```python
from build123d import *

# Parameters (mm, degrees)
F0_W      = 127
F0_H      = 127
F1_DEPTH  = 127
F2_R      = 10.16
F3_R      = 11.0292636168
F4_DEPTH  = 5.08
F6_DEPTH  = 5.08
F7_R      = 8.89
F8_DEPTH  = 5.08
F9_R      = 11.176
F10_DEPTH = 5.08
F12_DEPTH = 5.08
F14_DEPTH = 5.08


with BuildPart() as f1:
    # F0 (on Top) → F1 (new body)
    with BuildSketch(Plane.XY):
        with Locations((-72.0648214515, 42.2182492242)):
            Rectangle(F0_W, F0_H)
    extrude(amount=F1_DEPTH)

    # F2
    f2_edges = [f1.edges().sort_by_distance(p)[0] for p in [
        (-135.564821, -21.281751, 63.5),
        (-8.564821, -21.281751, 63.5),
        (-72.064821, -21.281751, 0),
        (-72.064821, -21.281751, 127),
        (-72.064821, 105.718249, 127),
        (-135.564821, 42.218249, 127),
        (-8.564821, 42.218249, 127),
        (-135.564821, 105.718249, 63.5),
        (-135.564821, 42.218249, 0),
        (-8.564821, 105.718249, 63.5),
        (-72.064821, 105.718249, 0),
        (-8.564821, 42.218249, 0),
    ]]
    fillet(f2_edges, radius=F2_R)

    # F3 (on face) → F4 (cut)
    with BuildSketch(Plane(origin=(0, 0, 0), x_dir=(1, 0, 0), z_dir=(0, 0, -1))):
        with Locations((-72.0648214515, -42.2182492242)):
            Circle(F3_R)
    extrude(amount=-F4_DEPTH, mode=Mode.SUBTRACT)

    # F5 (on face) → F6 (cut)
    with BuildSketch(Plane.XY.offset(127)):
        with BuildLine():
            Line((-100.0048214515, 61.2682492242), (-100.0048214515, 79.0482492242))
            ThreePointArc((-100.0048214515, 79.0482492242), (-108.8948214515, 70.1582492242), (-100.0048214515, 61.2682492242))
        make_face()
        with BuildLine():
            ThreePointArc((-91.1148214515, 70.1582492242), (-93.7186421668, 76.444428509), (-100.0048214515, 79.0482492242))
            Line((-100.0048214515, 79.0482492242), (-100.0048214515, 61.2682492242))
            ThreePointArc((-100.0048214515, 61.2682492242), (-93.7186421668, 63.8720699395), (-91.1148214515, 70.1582492242))
        make_face()
        with BuildLine():
            ThreePointArc((-100.0048214515, 53.6482492242), (-108.8948214515, 44.7582492242), (-100.0048214515, 35.8682492242))
            Line((-100.0048214515, 35.8682492242), (-100.0048214515, 53.6482492242))
        make_face()
        with BuildLine():
            Line((-100.0048214515, 53.6482492242), (-100.0048214515, 35.8682492242))
            ThreePointArc((-100.0048214515, 35.8682492242), (-93.7186421668, 38.4720699395), (-91.1148214515, 44.7582492242))
            ThreePointArc((-91.1148214515, 44.7582492242), (-93.7186421668, 51.044428509), (-100.0048214515, 53.6482492242))
        make_face()
        with BuildLine():
            Line((-44.1248214515, 61.2682492242), (-44.1248214515, 79.0482492242))
            ThreePointArc((-44.1248214515, 79.0482492242), (-53.0148214515, 70.1582492242), (-44.1248214515, 61.2682492242))
        make_face()
        with BuildLine():
            ThreePointArc((-35.2348214515, 70.1582492242), (-37.8386421668, 76.444428509), (-44.1248214515, 79.0482492242))
            Line((-44.1248214515, 79.0482492242), (-44.1248214515, 61.2682492242))
            ThreePointArc((-44.1248214515, 61.2682492242), (-37.8386421668, 63.8720699395), (-35.2348214515, 70.1582492242))
        make_face()
        with BuildLine():
            ThreePointArc((-44.1248214515, 53.6482492242), (-53.0148214515, 44.7582492242), (-44.1248214515, 35.8682492242))
            Line((-44.1248214515, 35.8682492242), (-44.1248214515, 53.6482492242))
        make_face()
        with BuildLine():
            Line((-44.1248214515, 53.6482492242), (-44.1248214515, 35.8682492242))
            ThreePointArc((-44.1248214515, 35.8682492242), (-37.8386421668, 38.4720699395), (-35.2348214515, 44.7582492242))
            ThreePointArc((-35.2348214515, 44.7582492242), (-37.8386421668, 51.044428509), (-44.1248214515, 53.6482492242))
        make_face()
        with BuildLine():
            ThreePointArc((-100.0048214515, 28.2482492242), (-108.8948214515, 19.3582492242), (-100.0048214515, 10.4682492242))
            Line((-100.0048214515, 10.4682492242), (-100.0048214515, 28.2482492242))
        make_face()
        with BuildLine():
            Line((-100.0048214515, 28.2482492242), (-100.0048214515, 10.4682492242))
            ThreePointArc((-100.0048214515, 10.4682492242), (-93.7186421668, 13.0720699395), (-91.1148214515, 19.3582492242))
            ThreePointArc((-91.1148214515, 19.3582492242), (-93.7186421668, 25.644428509), (-100.0048214515, 28.2482492242))
        make_face()
        with BuildLine():
            ThreePointArc((-44.1248214515, 28.2482492242), (-53.0148214515, 19.3582492242), (-44.1248214515, 10.4682492242))
            Line((-44.1248214515, 10.4682492242), (-44.1248214515, 28.2482492242))
        make_face()
        with BuildLine():
            Line((-44.1248214515, 28.2482492242), (-44.1248214515, 10.4682492242))
            ThreePointArc((-44.1248214515, 10.4682492242), (-37.8386421668, 13.0720699395), (-35.2348214515, 19.3582492242))
            ThreePointArc((-35.2348214515, 19.3582492242), (-37.8386421668, 25.644428509), (-44.1248214515, 28.2482492242))
        make_face()
    extrude(amount=-F6_DEPTH, mode=Mode.SUBTRACT)

    # F7 (on face) → F8 (cut)
    with BuildSketch(Plane(origin=(-135.5648214515, 0, 0), x_dir=(0, -1, 0), z_dir=(-1, 0, 0))):
        with Locations((-68.8882492242, 90.17)):
            Circle(F7_R)
        with Locations((-68.8882492242, 36.83)):
            Circle(F7_R)
        with Locations((-15.5482492242, 36.83)):
            Circle(F7_R)
        with Locations((-15.5482492242, 90.17)):
            Circle(F7_R)
    extrude(amount=-F8_DEPTH, mode=Mode.SUBTRACT)

    # F9 (on face) → F10 (cut)
    with BuildSketch(Plane.YZ.offset(-8.5648214515)):
        with Locations((6.6322155756, 99.0860336486)):
            Circle(F9_R)
        with Locations((77.8042828729, 27.9139663514)):
            Circle(F9_R)
        with Locations((42.2182492242, 63.5)):
            Circle(F9_R)
    extrude(amount=-F10_DEPTH, mode=Mode.SUBTRACT)

    # F11 (on face) → F12 (cut)
    with BuildSketch(Plane.XZ.offset(21.2817507758)):
        with BuildLine():
            ThreePointArc((-99.8604116578, 102.4715902063), (-106.7595416177, 112.7968678616), (-118.9390370444, 110.3742155928))
            Line((-118.9390370444, 110.3742155928), (-103.1337862713, 94.5689648197))
            ThreePointArc((-103.1337862713, 94.5689648197), (-100.7111340025, 98.1947201662), (-99.8604116578, 102.4715902063))
        make_face()
        with BuildLine():
            ThreePointArc((-40.9958566318, 32.4310351803), (-40.9958566318, 16.6257844072), (-25.1906058587, 16.6257844072))
            Line((-25.1906058587, 16.6257844072), (-40.9958566318, 32.4310351803))
        make_face()
        with BuildLine():
            Line((-40.9958566318, 32.4310351803), (-25.1906058587, 16.6257844072))
            ThreePointArc((-25.1906058587, 16.6257844072), (-22.7679535899, 20.2515397536), (-21.9172312452, 24.5284097937))
            ThreePointArc((-21.9172312452, 24.5284097937), (-28.8163612051, 34.8536874491), (-40.9958566318, 32.4310351803))
        make_face()
        with BuildLine():
            ThreePointArc((-103.1337862713, 32.4310351803), (-118.9390370444, 32.4310351803), (-118.9390370444, 16.6257844072))
            Line((-118.9390370444, 16.6257844072), (-103.1337862713, 32.4310351803))
        make_face()
        with BuildLine():
            Line((-103.1337862713, 32.4310351803), (-118.9390370444, 16.6257844072))
            ThreePointArc((-118.9390370444, 16.6257844072), (-106.7595416177, 14.2031321384), (-99.8604116578, 24.5284097937))
            ThreePointArc((-99.8604116578, 24.5284097937), (-100.7111340025, 28.8052798338), (-103.1337862713, 32.4310351803))
        make_face()
        with BuildLine():
            ThreePointArc((-64.162196065, 71.4026253865), (-72.0648214515, 74.676), (-79.9674468381, 71.4026253865))
            Line((-79.9674468381, 71.4026253865), (-72.0648214515, 63.5))
            Line((-72.0648214515, 63.5), (-64.162196065, 71.4026253865))
        make_face()
        with BuildLine():
            Line((-72.0648214515, 63.5), (-79.9674468381, 71.4026253865))
            ThreePointArc((-79.9674468381, 71.4026253865), (-83.2408214515, 63.5), (-79.9674468381, 55.5973746135))
            Line((-79.9674468381, 55.5973746135), (-72.0648214515, 63.5))
        make_face()
        with BuildLine():
            Line((-64.162196065, 71.4026253865), (-72.0648214515, 63.5))
            Line((-72.0648214515, 63.5), (-64.162196065, 55.5973746135))
            ThreePointArc((-64.162196065, 55.5973746135), (-61.7395437962, 59.2231299599), (-60.8888214515, 63.5))
            ThreePointArc((-60.8888214515, 63.5), (-61.7395437962, 67.7768700401), (-64.162196065, 71.4026253865))
        make_face()
        with BuildLine():
            Line((-64.162196065, 55.5973746135), (-72.0648214515, 63.5))
            Line((-72.0648214515, 63.5), (-79.9674468381, 55.5973746135))
            ThreePointArc((-79.9674468381, 55.5973746135), (-72.0648214515, 52.324), (-64.162196065, 55.5973746135))
        make_face()
        with BuildLine():
            Line((-103.1337862713, 94.5689648197), (-118.9390370444, 110.3742155928))
            ThreePointArc((-118.9390370444, 110.3742155928), (-118.9390370444, 94.5689648197), (-103.1337862713, 94.5689648197))
        make_face()
        with BuildLine():
            Line((-40.9958566318, 94.5689648197), (-25.1906058587, 110.3742155928))
            ThreePointArc((-25.1906058587, 110.3742155928), (-40.9958566318, 110.3742155928), (-40.9958566318, 94.5689648197))
        make_face()
        with BuildLine():
            ThreePointArc((-21.9172312452, 102.4715902063), (-22.7679535899, 106.7484602464), (-25.1906058587, 110.3742155928))
            Line((-25.1906058587, 110.3742155928), (-40.9958566318, 94.5689648197))
            ThreePointArc((-40.9958566318, 94.5689648197), (-28.8163612051, 92.1463125509), (-21.9172312452, 102.4715902063))
        make_face()
    extrude(amount=-F12_DEPTH, mode=Mode.SUBTRACT)

    # F13 (on face) → F14 (cut)
    with BuildSketch(Plane(origin=(0, 105.7182492242, 0), x_dir=(-1, 0, 0), z_dir=(0, 1, 0))):
        with BuildLine():
            ThreePointArc((90.875736666, 44.6890847855), (90.875736666, 28.8838340124), (106.6809874391, 28.8838340124))
            Line((106.6809874391, 28.8838340124), (90.875736666, 44.6890847855))
        make_face()
        with BuildLine():
            ThreePointArc((37.448655464, 98.1161659876), (37.448655464, 82.3109152145), (53.253906237, 82.3109152145))
            Line((53.253906237, 82.3109152145), (37.448655464, 98.1161659876))
        make_face()
        with BuildLine():
            Line((37.448655464, 98.1161659876), (53.253906237, 82.3109152145))
            ThreePointArc((53.253906237, 82.3109152145), (55.6765585058, 85.9366705609), (56.5272808505, 90.213540601))
            ThreePointArc((56.5272808505, 90.213540601), (49.6281508906, 100.5388182564), (37.448655464, 98.1161659876))
        make_face()
        with BuildLine():
            Line((90.875736666, 44.6890847855), (106.6809874391, 28.8838340124))
            ThreePointArc((106.6809874391, 28.8838340124), (109.1036397079, 32.5095893589), (109.9543620526, 36.786459399))
            ThreePointArc((109.9543620526, 36.786459399), (103.0552320927, 47.1117370543), (90.875736666, 44.6890847855))
        make_face()
    extrude(amount=-F14_DEPTH, mode=Mode.SUBTRACT)


solid = f1.part
```
Source: CAD feature listing. Evaluate the final solid. Frame: model axes, mm. A direction names the side the tool comes from. Coordinates: 2 decimals unless noted, no trailing zeros. Write each loop counter-clockwise with the first axis right and the second up, starting at its lowest first coordinate (ties: lowest second). Pieces come first, ordered by that corner, then holes. Notation, with made-up numbers: (42.25, 20.25) -> (88.25, 20.25) arc R33 cw to (88.25, 56.25) -> close; hole circle Ø3 at (27.25, 79.25). An arc over 180 degrees is marked (long way). Return JSON: item names as keys, results as strings. Group by question number.
1) Set-up query: faces 4 (the face through (-133.06, 77.77, 37.22)), 5 (the face through (-100, 19, 121.92)), 6 (the face through (-72, -16.202, 64)), 7 (the face through (-13.645, 6, 99)). Return all of +Z, -Z, +X, -X, +Y, -Y with unobstructed straight access to the full face (end or side cutting, diameter ignored); none if empty.
2) Ray query, line 1 along X through (y, z) = (73, 84.5); line 2 along X through (y, z) = (-2.5, 95); line 3 along Z through (x, y) = (-18.5, 30.5). Return the intervals inside material, ascending.
3) Contact query for flat-ended pins moving along their axis: P1, Ø9, axis at x = -96, y = 71, coming from the +Z side; P2, Ø9, axis at y = 66.5, z = 37, coming from the -X side; P3, Ø6.5, axis at y = 6, z = 99.5, coming from the +X side. Output: stop coordinate, or through.
4) Section query D-D, the plane z = 41. Return loops of the section in (x, y).
5) Section query B-B, the plane z = 21. Return loops of the section in (x, y), plus the area to 3 significant figures.
6) Section query A-A, the plane y = 38. Return loops of the section in (x, z).
7) Mould query, pull axis Z, two halves, no side actions, for faces 1 (the face through (-85, 43, 0)), 2 (the face through (-132.67, 102.66, 64.25)), 3 (the face through (-13.645, 78, 28)). Classes: +Z half, -Z half, draft (parallel to the pull), parting line (faces both ways), or undercut.
8) Section query C-C, the plane x = -95.5. Return loops of the section in (y, z), plus the area to 3 significant figures.
From the geometry:
{
 "1": {"face 4": "-X", "face 5": "+Z", "face 6": "-Y", "face 7": "+X"},
 "2": {"line 1": "-130.48 to -8.56", "line 2": "-135.56 to -13.64", "line 3": "0 to 127"},
 "3": {"P1": "z = 121.92", "P2": "x = -130.48", "P3": "x = -13.64"},
 "4": {"outline": "(-135.56, -11.12) arc R10.16 ccw to (-125.4, -21.28) -> (-18.72, -21.28) arc R10.16 ccw to (-8.56, -11.12) -> (-8.56, 95.56) arc R10.16 ccw to (-18.72, 105.72) -> (-88.43, 105.72) -> (-88.43, 100.64) -> (-109.13, 100.64) -> (-109.13, 105.72) -> (-125.4, 105.72) arc R10.16 ccw to (-135.56, 95.56) -> (-135.56, 76.74) -> (-130.48, 76.74) -> (-130.48, 61.04) -> (-135.56, 61.04) -> (-135.56, 23.4) -> (-130.48, 23.4) -> (-130.48, 7.7) -> (-135.56, 7.7) -> close"},
 "5": {"outline": "(-135.56, -11.12) arc R10.16 ccw to (-125.4, -21.28) -> (-121.64, -21.28) -> (-121.64, -16.2) -> (-100.43, -16.2) -> (-100.43, -21.28) -> (-43.7, -21.28) -> (-43.7, -16.2) -> (-22.49, -16.2) -> (-22.49, -21.28) -> (-18.72, -21.28) arc R10.16 ccw to (-8.56, -11.12) -> (-8.56, 69.02) -> (-13.64, 69.02) -> (-13.64, 86.58) -> (-8.56, 86.58) -> (-8.56, 95.56) arc R10.16 ccw to (-18.72, 105.72) -> (-125.4, 105.72) arc R10.16 ccw to (-135.56, 95.56) -> close", "area": "15,700 mm²"},
 "6": {"outline": "(-135.56, 10.16) arc R10.16 ccw to (-125.4, 0) -> (-82.26, 0) -> (-82.26, 5.08) -> (-61.87, 5.08) -> (-61.87, 0) -> (-18.72, 0) arc R10.16 ccw to (-8.56, 10.16) -> (-8.56, 53.15) -> (-13.64, 53.15) -> (-13.64, 73.85) -> (-8.56, 73.85) -> (-8.56, 116.84) arc R10.16 ccw to (-18.72, 127) -> (-38.35, 127) -> (-38.35, 121.92) -> (-49.9, 121.92) -> (-49.9, 127) -> (-94.23, 127) -> (-94.23, 121.92) -> (-105.78, 121.92) -> (-105.78, 127) -> (-125.4, 127) arc R10.16 ccw to (-135.56, 116.84) -> close"},
 "7": {"face 1": "-Z half", "face 2": "draft", "face 3": "undercut"},
 "8": {"outline": "(-21.28, 10.16) arc R10.16 ccw to (-11.12, 0) -> (95.56, 0) arc R10.16 ccw to (105.72, 10.16) -> (105.72, 26.1) -> (100.64, 26.1) -> (100.64, 47.47) -> (105.72, 47.47) -> (105.72, 116.84) arc R10.16 ccw to (95.56, 127) -> (77.82, 127) -> (77.82, 121.92) -> (62.49, 121.92) -> (62.49, 127) -> (52.42, 127) -> (52.42, 121.92) -> (37.09, 121.92) -> (37.09, 127) -> (27.02, 127) -> (27.02, 121.92) -> (11.69, 121.92) -> (11.69, 127) -> (-11.12, 127) arc R10.16 ccw to (-21.28, 116.84) -> close", "area": "15,700 mm²"}
}
